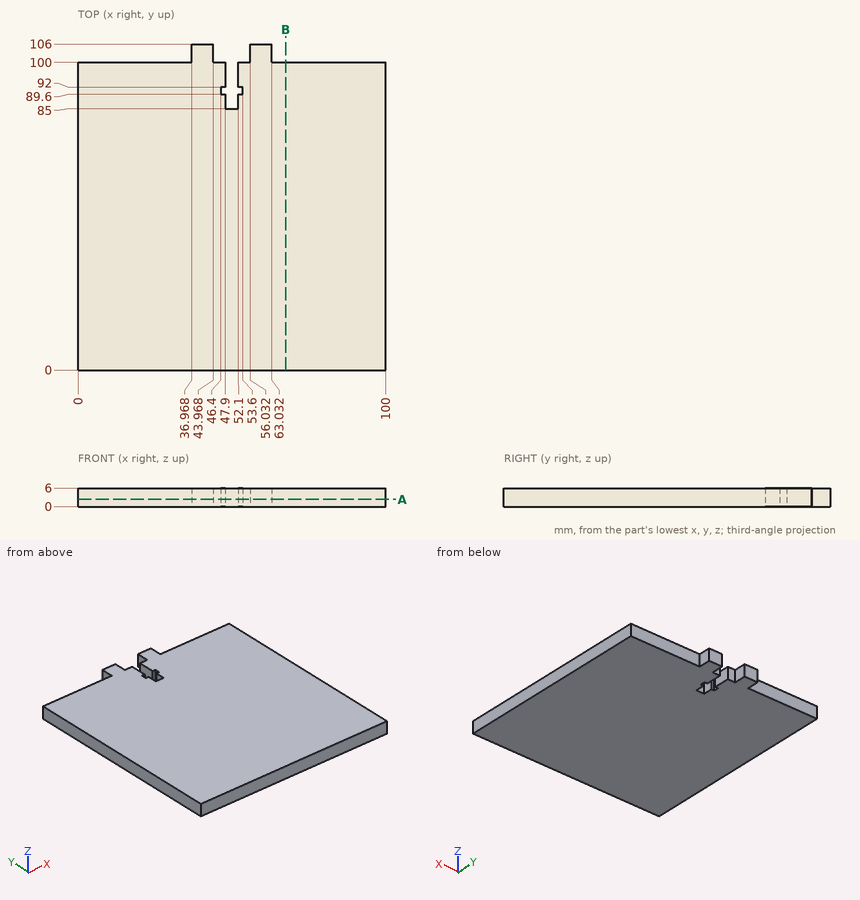
Design review of the part shown in the three views and the two pictorial views. Dimensions are in mm from the part's minimum x, y and z. Coordinates: 2 decimals unless noted, no trailing zeros. Order: outer loops, then holes, each group sorted by start corner. A loop starts at its lowest first (then second) coordinate and runs counter-clockwise, first axis right, second up. Notation, with made-up numbers: (86, -3) -> (126, -3) arc R11 cw to (126, 17) -> close; hole circle Ø6 at (73.5, 78.25). An arc over 180 degrees is marked (long way). Use one line per item in the form item = value. Start each with the question number.
(1) Add section A-A on z = 2.4. State the section outline as (x, y) points.
(2) For probe 1 along X at (y, z) = (88.5, 2.5); probe 2 along Y at (x, z) = (94, 4); probe 3 along Y at (x, z) = (51, 4.15), list the stretches that pass through material, from the lowest coordinate up.
(3) Insertion check: pin 1 (1.8 mm diameter, centred on y = 102.5, z = 2.5, fed in from +X); pin 2 (0.5 mm diameter, centred on x = 53, z = 2, fed in from +Y); pin 3 (1.8 mm diameter, centred on y = 103, z = 3.5, fed in from -X). Each pin has a flat end and moves straight along its axis. Give the tip position at first contact, or say it passes through.
(4) Add section B-B on x = 67.5. State the section outline as (y, z) points.
Answer block:
q1.outline = (0, 0) -> (100, 0) -> (100, 100) -> (63.03, 100) -> (63.03, 106) -> (56.03, 106) -> (56.03, 100) -> (52.1, 100) -> (52.1, 92) -> (53.6, 92) -> (53.6, 89.6) -> (52.1, 89.6) -> (52.1, 85) -> (47.9, 85) -> (47.9, 89.6) -> (46.4, 89.6) -> (46.4, 92) -> (47.9, 92) -> (47.9, 100) -> (43.97, 100) -> (43.97, 106) -> (36.97, 106) -> (36.97, 100) -> (0, 100) -> close
q2.probe_1 = 0 to 47.9, 52.1 to 100
q2.probe_2 = 0 to 100
q2.probe_3 = 0 to 85
q3.pin_1 = 63.03
q3.pin_2 = 100
q3.pin_3 = 36.97
q4.outline = (0, 0) -> (100, 0) -> (100, 6) -> (0, 6) -> close
